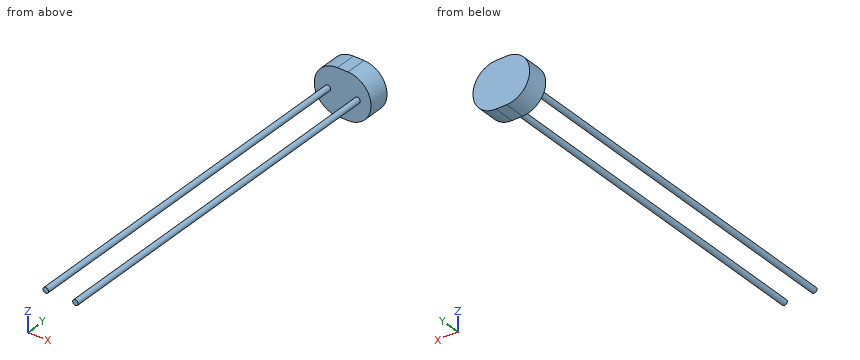
from build123d import *

# Parameters (mm, degrees)
SALIENTE_EXTRUIR1_DEPTH = 1.9
CROQUIS3_R              = 0.25
SALIENTE_EXTRUIR2_DEPTH = 33.4


with BuildPart() as part:
    # Croquis1 → Saliente-Extruir1 (new body)
    with BuildSketch(Plane(origin=(0, 0, 0), x_dir=(1, 0, 0), z_dir=(0, 1, 0))):
        with BuildLine():
            Line((-0.475, 2.075), (0.475, 2.075))
            ThreePointArc((0.475, 2.075), (2.55, 0), (0.475, -2.075))
            Line((0.475, -2.075), (-0.475, -2.075))
            ThreePointArc((-0.475, -2.075), (-2.55, 0), (-0.475, 2.075))
        make_face()
    extrude(amount=SALIENTE_EXTRUIR1_DEPTH)

    # Croquis3 → Saliente-Extruir2 (add)
    with BuildSketch(Plane.XZ):
        with Locations(Location((-1.333712644, 0, 0), (0, 0, 90))):
            Circle(CROQUIS3_R)
        with Locations(Location((1.333712644, 0, 0), (0, 0, 90))):
            Circle(CROQUIS3_R)
    extrude(amount=SALIENTE_EXTRUIR2_DEPTH)


solid = part.part
Here's how the part is built. I have some questions about the finished solid (model axes, mm). Coordinates: 2 decimals unless noted, no trailing zeros. Write each loop counter-clockwise with the first axis right and the second up, starting at its lowest first coordinate (ties: lowest second). Pieces come first, ordered by that corner, then holes.
1) I'm going to push flat-ended pins straight in: pin 1 (1.5 mm diameter, centred on x = 1.5, y = -17, fed in from -Z); pin 2 (1 mm diameter, centred on y = -26, z = 0, fed in from +X). Where does each tip first touch, or does it pass through?
Filled in:
pin 1: stops at z = -0.25
pin 2: stops at x = 1.58
2) If we section it at A-A (y = -16.5): List the corners of the cut face in (x, z) for me.
Filled in:
outline: circle Ø0.5 at (-1.33, 0); circle Ø0.5 at (1.33, 0)
3) If we section it at C-C (x = -2): List the corners of the cut face in (y, z) for me, plus the area to 3 significant figures.
Filled in:
outline: (0, -1.41) - (1.9, -1.41) - (1.9, 1.41) - (0, 1.41) - close
area: 5.35 mm2
4) If we section it at B-B (z = 1.7): List the corners of the cut face in (x, y) for me, plus the area to 3 significant figures.
Filled in:
outline: (-1.66, 0) - (1.66, 0) - (1.66, 1.9) - (-1.66, 1.9) - close
area: 6.33 mm2
5) If I drill on line 1 (Y direction, x = 1.75, z = -0.2); line 2 (X direction, y = -3.5, z = -0.15); line 3 (Z direction, x = -1.5, y = -12), over which ranges is the centre line in solid material (lowest first)?
Filled in:
line 1: y = 0 to 1.9
line 2: x = -1.53 to -1.13, 1.13 to 1.53
line 3: z = -0.19 to 0.19
